Answer from the drawing. Dimensions are ordinates in mm from the lowest x, y and z of the part. Coordinates: 2 decimals unless noted, no trailing zeros. Loops run counter-clockwise (first coordinate to the right, second up) from the corner with the lowest first, then second, coordinate; pieces in that order, holes last. Notation, with made-up numbers: M 51,86.25 L 57,86.25 A30 ccw 57,118.25 Z; hole C 33.5,-7 d3. An arc over 180 degrees is marked long. Answer as CSV lines item,"result". Start each with the question number.
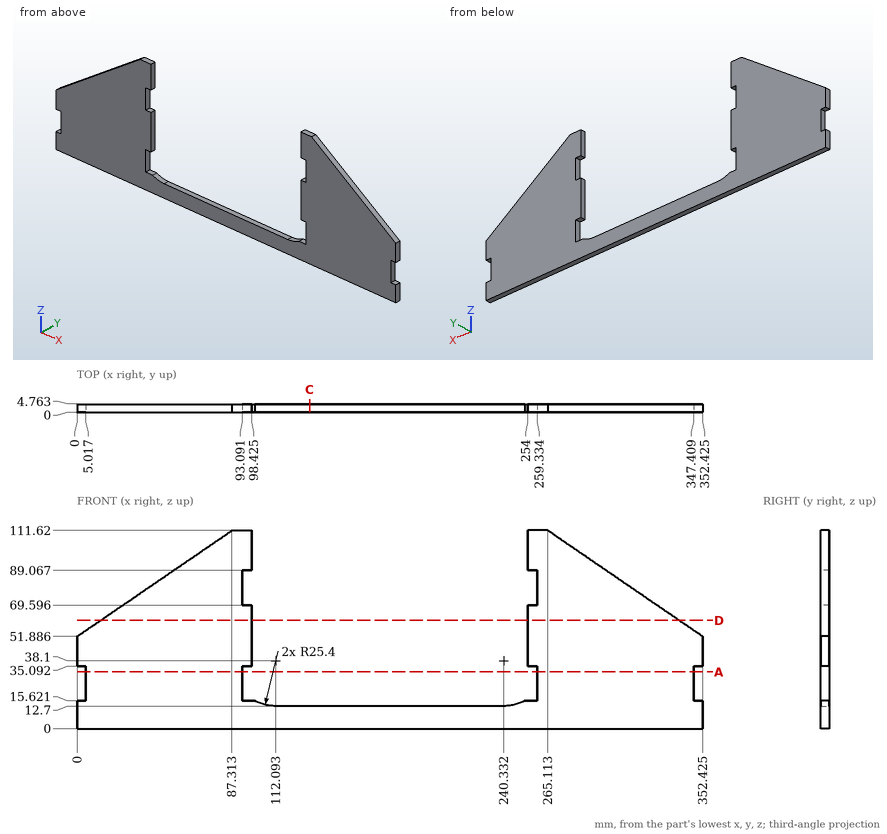
Item 1: Section D-D on z = 61 is taken. Determine the outline of the cut face in (x, y) (1 decimal).
Item 2: Each of these flat-tipped pins is pushed along its axis until it touches: P1, Ø1.5, axis at x = 98.5, z = 94.5, coming from the +Y side; P2, Ø1.4, axis at y = 3, z = 105.5, coming from the +X side; P3, Ø1.4, axis at x = 197.5, y = 3.5, coming from the +Z side. Where does it stop, or does it pass through?
Item 3: Section C-C on x = 131 is taken. Determine the outline of the cut face in (y, z).
Item 4: Consider line 1 (Z direction, x = 96, y = 1.1) (1 decimal); line 2 (X direction, y = 0.45, z = 21) (1 decimal); line 3 (X direction, y = 1.45, z = 45) (1 decimal). Determine where each line is inside the solid, lowest interval first.
Item 5: Section A-A on z = 32 is taken. Determine the outline of the cut face in (x, y) (1 decimal).
Results are:
1,outline,"M 13.3,0 L 98.4,0 L 98.4,4.8 L 13.3,4.8 Z; M 254,0 L 339.1,0 L 339.1,4.8 L 254,4.8 Z"
2,P1,"y = 4.76"
2,P2,"x = 275.08"
2,P3,"z = 12.7"
3,outline,"M 0,0 L 4.76,0 L 4.76,12.7 L 0,12.7 Z"
4,line 1,"0 to 15.6, 35.1 to 69.6, 89.1 to 111.6"
4,line 2,"5 to 93.1, 259.3 to 347.4"
4,line 3,"0 to 98.4, 254 to 352.4"
5,outline,"M 5,0 L 93.1,0 L 93.1,4.8 L 5,4.8 Z; M 259.3,0 L 347.4,0 L 347.4,4.8 L 259.3,4.8 Z"
